Build history of the part. All positions in model axes, mm. Round coordinates to 2 decimals unless told otherwise and drop trailing zeros. Write each loop counter-clockwise with the first axis right and the second up, starting at its lowest first coordinate (ties: lowest second). Pieces come first, ordered by that corner, then holes.
1) Flat gauge pin, fed straight in: pin 1 (5.5 mm diameter, centred on x = 25.4, z = -53.975, fed in from +Y). Where does the tip first touch, or does it go through?
2) Pull direction Z, two halves, no side cores. Call faces 1 (the cylindrical face through (33.97, 1.61, 65.77)), 2 (the flat face through (0, 2, -66.675)), 3 (the cylindrical face through (-24.96, 1.565, 50.626)): +Z half, -Z half, draft (parallel to the pull), parting line (faces both ways), or undercut.
3) Wall check: probe 1 along X at (y, z) = (1.3, 0) (3 decimals); probe 2 along X at (y, z) = (2.75, 51.5) (3 decimals); probe 3 along Z at (x, y) = (25, 1.9) (3 decimals). Give the ranges that are in metal, low to high.
4) Saw through at C-C (y = 1.35). State how many separate pieces and enclosed holes the cut face has, plus the area to 3 significant figures.
5) Saw through at A-A (z = 0). Write the cut outline in (x, y) (3 decimals).
6) Saw through at B-B (x = 0). Write the cut outline in (y, z) (3 decimals), plus the area to 3 significant figures.
7) Saw through at D-D (x = -25.4). Write the cut outline in (y, z) (3 decimals), plus the area to 3 significant figures.
from build123d import *

# Parameters (mm, degrees)
SKETCH1_W                      = 69.85
SKETCH1_H                      = 133.35
BOSS_EXTRUDE1_DEPTH            = 3.175
SKETCH2_R                      = 30
CUT_EXTRUDE1_DEPTH             = 3.175
F_3_16_0_1875_DIAMETER_HOLE1_D = 4.7625
F_1_4_CLEARANCE_HOLE1_D        = 6.7564
F_1_4_CLEARANCE_HOLE1_DEPTH    = 3.175
FILLET1_R                      = 3.175


with BuildPart() as part:
    # Sketch1 → Boss-Extrude1 (new body)
    with BuildSketch(Plane(origin=(0, 0, 0), x_dir=(1, 0, 0), z_dir=(0, 1, 0))):
        Rectangle(SKETCH1_W, SKETCH1_H)
    extrude(amount=BOSS_EXTRUDE1_DEPTH)

    # Sketch2 → Cut-Extrude1 (cut)
    with BuildSketch(Plane(origin=(0, 3.175, 0), x_dir=(1, 0, 0), z_dir=(0, 1, 0))):
        with Locations(Location((0, 0, 0), (0, 0, 270))):
            Circle(SKETCH2_R)
    extrude(amount=-CUT_EXTRUDE1_DEPTH, mode=Mode.SUBTRACT)

    # 3/16 (0.1875) Diameter Hole1 (through all)
    with Locations(Plane(origin=(0, 3.175, 0), x_dir=(1, 0, 0), z_dir=(0, 1, 0))):
        with Locations((25, -25), (25, 25), (-25, -25), (-25, 25)):
            Hole(F_3_16_0_1875_DIAMETER_HOLE1_D / 2)

    # 1/4 Clearance Hole1
    with Locations(Plane(origin=(0, 3.175, 0), x_dir=(1, 0, 0), z_dir=(0, 1, 0))):
        with Locations((0, 0), (25.4, 53.975), (-25.4, -53.975), (-25.4, 53.975), (25.4, -53.975)):
            Hole(F_1_4_CLEARANCE_HOLE1_D / 2, depth=F_1_4_CLEARANCE_HOLE1_DEPTH)

    # Fillet1
    fillet1_edges = [part.edges().sort_by_distance(p)[0] for p in [
        (34.925, 1.5875, 66.675),
        (-34.925, 1.5875, 66.675),
        (-34.925, 1.5875, -66.675),
        (34.925, 1.5875, -66.675),
    ]]
    fillet(fillet1_edges, radius=FILLET1_R)


solid = part.part
Evaluation:
1. pin 1: passes through
2. face 1: +Z half
2. face 2: -Z half
2. face 3: undercut
3. probe 1: x = -34.925 to -30, 30 to 34.925
3. probe 2: x = -34.925 to -27.699, -23.101 to 23.101, 27.699 to 34.925
3. probe 3: z = -66.675 to -57.329, -50.621 to -27.381, -22.619 to -16.583, 16.583 to 22.619, 27.381 to 50.621, 57.329 to 66.675
4. separate pieces: 1
4. enclosed holes: 9
4. area: 6,260 mm2
5. outline: (-34.925, 0) - (-30, 0) - (-30, 3.175) - (-34.925, 3.175) - close; (30, 0) - (34.925, 0) - (34.925, 3.175) - (30, 3.175) - close
6. outline: (0, -66.675) - (3.175, -66.675) - (3.175, -30) - (0, -30) - close; (0, 30) - (3.175, 30) - (3.175, 66.675) - (0, 66.675) - close
6. area: 233 mm2
7. outline: (0, -66.675) - (3.175, -66.675) - (3.175, -57.353) - (0, -57.353) - close; (0, -50.597) - (3.175, -50.597) - (3.175, -27.347) - (0, -27.347) - close; (0, -22.653) - (3.175, -22.653) - (3.175, -15.964) - (0, -15.964) - close; (0, 15.964) - (3.175, 15.964) - (3.175, 22.653) - (0, 22.653) - close; (0, 27.347) - (3.175, 27.347) - (3.175, 50.597) - (0, 50.597) - close; (0, 57.353) - (3.175, 57.353) - (3.175, 66.675) - (0, 66.675) - close
7. area: 249 mm2
